Autodesk Inventor part; units mm, degrees
ref_plane "Pracovní rovina1" through (-500, -4173.9622, 0) normal (1, 0, 0) x (0, 1, 0)
ref_plane "YZ Plane" through (0, 0, 0) normal (1, 0, 0) x (0, 1, 0)
ref_plane "XZ Plane" through (0, 0, 0) normal (0, 1, 0) x (-1, 0, 0)
sketch "Náčrt1" plane through (0, 0, 0) normal (0, 0, 1) x (1, 0, 0)
  line L0 (-500, -500) -> (500, -500)
  line L1 (500, -500) -> (500, 500)
  line L2 (500, 500) -> (-500, 500)
  line L3 (-500, 500) -> (-500, -500)
  line L4 (-500, -500) -> (500, 500) construction
  line L5 (500, -500) -> (-500, 500) construction
  circle A0 centre (0, 0) radius 400
  dimension "d0" = 1000
  dimension "d1" = 1000
  dimension "d6" = 800
extrude "Vysunutí1" add sketch "Náčrt1" along normal blind 500
sketch "Náčrt2" plane through (500, -500, 0) normal (1, 0, 0) x (0, 0, -1)
  line L0 (-500, 0) -> (-500, 1000)
  line L1 (-500, 500) -> (-400, 500)
  line L2 (-400, 500) -> (-500, 400)
  point P0 (0, 500)
  dimension "d7" = 100
  dimension "d8" = 45
ref_plane "Pracovní rovina1" through (-500, -4173.9622, 0) normal (1, 0, 0) x (0, 1, 0)
extrude "Vysunutí2" cut sketch "Náčrt2" against normal up to surface (1000 mm away)
equation "\"d1\" = d0"
properties part number "B2-Y"
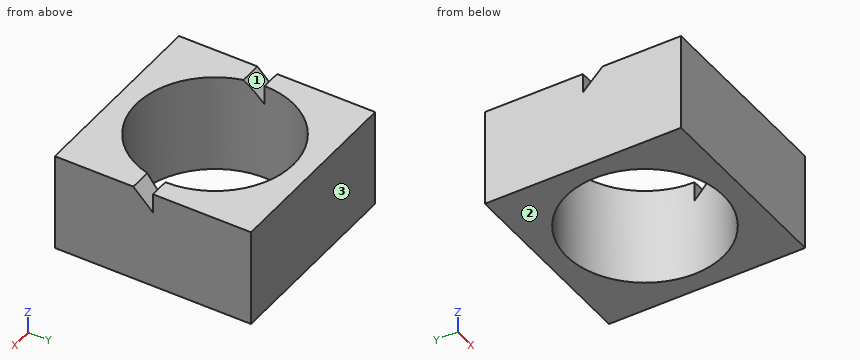
Geometry: final body of the model. Coordinates: model frame, mm. Face numbers are marked on the shaded views. Round coordinates to 2 decimals unless told otherwise and drop trailing zeros. Order: outer loops, then holes, each group sorted by start corner. A loop starts at its lowest first (then second) coordinate and runs counter-clockwise, first axis right, second up. Notation, with made-up numbers: (14, 56) -> (27, 56) arc R19 ccw to (27, 72) -> close; hole circle Ø5 at (54, 6). An arc over 180 degrees is marked (long way). Write each question's results on one line, items separated by ' | '.
Q1. Section query A-A (x = 0). Output: boundary loops of the cut face in (y, z), and give its area (3 significant figures).
Response values:
outline: (-500, 0) -> (-400, 0) -> (-400, 500) -> (-500, 500) -> close; (400, 0) -> (500, 0) -> (500, 500) -> (400, 500) -> close | area: 100,000 mm²
Q2. Section query B-B (y = 300.5). Output: boundary loops of the cut face in (x, z), and give its area (3 significant figures).
Response values:
outline: (-500, 0) -> (-264.01, 0) -> (-264.01, 500) -> (-500, 500) -> close; (264.01, 0) -> (500, 0) -> (500, 500) -> (264.01, 500) -> close | area: 236,000 mm²
Q3. Section query C-C (z = 458). Output: boundary loops of the cut face in (x, y), and give its area (3 significant figures).
Response values:
outline: (-500, -500) -> (500, -500) -> (500, -58) -> (395.77, -58) arc R400 cw to (-395.77, -58) -> (-500, -58) -> close; (-500, 0) -> (-400, 0) arc R400 cw to (400, 0) -> (500, 0) -> (500, 500) -> (-500, 500) -> close | area: 486,000 mm²
Q4. Pull-direction query (Y, two-part tool) for the marked faces 1, 2 and 3; classes: released by +Y, released by -Y, zero draft, split by the parting line, or undercut.
Response values:
face 1: undercut | face 2: zero draft | face 3: released by +Y
Q5. Section query D-D (z = 361). Output: boundary loops of the cut face in (x, y), and give its area (3 significant figures).
Response values:
outline: (-500, -500) -> (500, -500) -> (500, 500) -> (-500, 500) -> close; hole circle Ø800 at (0, 0) | area: 497,000 mm²
Q6. Ray query, line 1 along Y through (x, z) = (0, 194.5); line 2 along Y through (x, z) = (-99.5, 117.5). Return the intervals inside material, ascending.
Response values:
line 1: -500 to -400, 400 to 500 | line 2: -500 to -387.43, 387.43 to 500
